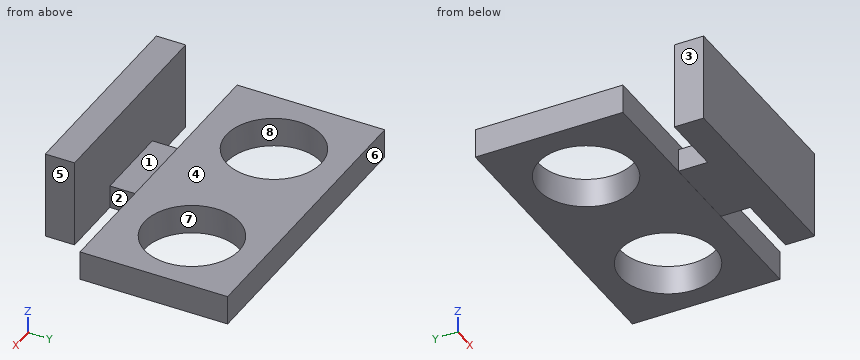
```python
from build123d import *

# Parameters (mm, degrees)
SKETCH1_W           = 35.5
SKETCH1_H           = 15
BOSS_EXTRUDE7_DEPTH = 5
SKETCH5_W           = 13.567085075
SKETCH5_H           = 3.932792286
BOSS_EXTRUDE8_DEPTH = 5
SKETCH6_W           = 50.2
SKETCH6_H           = 5
BOSS_EXTRUDE9_DEPTH = 25.2
SKETCH7_R           = 8.1
CUT_EXTRUDE1_DEPTH  = 10


with BuildPart() as part:
    # Sketch1 → Boss-Extrude7 (new body)
    with BuildSketch(Plane(origin=(0, 0, 0), x_dir=(1, 0, 0), z_dir=(0, 1, 0))):
        with Locations((32.254129859, 13.775388257)):
            Rectangle(SKETCH1_W, SKETCH1_H)
    extrude(amount=BOSS_EXTRUDE7_DEPTH)

    # Sketch5 → Boss-Extrude8 (add)
    with BuildSketch(Plane(origin=(0, 5, 0), x_dir=(1, 0, 0), z_dir=(0, 1, 0))):
        with Locations((31.950040022, 19.308992114)):
            Rectangle(SKETCH5_W, SKETCH5_H)
    extrude(amount=BOSS_EXTRUDE8_DEPTH)

    # Sketch6 → Boss-Extrude9 (add)
    with BuildSketch(Plane(origin=(1.124638213, 10, 0), x_dir=(1, 0, 0), z_dir=(0, 1, 0))):
        with Locations((31.402213384, 18.794771585)):
            Rectangle(SKETCH6_W, SKETCH6_H)
    extrude(amount=BOSS_EXTRUDE9_DEPTH)

    # Sketch7 → Cut-Extrude1 (cut)
    with BuildSketch(Plane.XY.offset(-16.294771585)):
        with Locations((19.758900119, 22.875876323)):
            Circle(SKETCH7_R)
        with Locations((45.958900119, 22.875876323)):
            Circle(SKETCH7_R)
    extrude(amount=-CUT_EXTRUDE1_DEPTH, mode=Mode.SUBTRACT)


solid = part.part
```
Geometry check sheet. Reference: the model listing, model coordinates, mm. Face numbers are marked on the shaded views. A direction names the side the tool comes from. Give positions to 0.01 mm unless a question says otherwise; leave off trailing zeros. Loops run counter-clockwise (first coordinate to the right, second up) from the corner with the lowest first, then second, coordinate; pieces in that order, holes last. Notation, with made-up numbers: M -8,57.5 L -4,57.5 A27 ccw -4,87.5 Z; hole C -15.75,81.5 d1. An arc over 180 degrees is marked long. Write item = value, one per line. Start each with the question number.
1. Section check A-A, the plane y = 30. Enter the section's corners in (x, z), plus the area to 3 significant figures.
2. Section check C-C, the plane x = 22.5. Enter the section's corners in (y, z).
3. Thickness scan on probe 1 along Y at (x, z) = (20, -16.75); probe 2 along Y at (x, z) = (41, -19.5); probe 3 along Y at (x, z) = (38, -7.25). Record the ranges inside material, lowest first.
4. Section check D-D, the plane z = -18. Enter the section's corners in (x, y), plus the area to 3 significant figures.
5. Tool access check on the marked faces 1, 2, 3 and 4. Record the directions out of +Z, -Z, +X, -X, +Y, -Y that give a thin tool (end or side, any length) a straight path to the whole face; none if there is none.
6. Draft check along X on the marked faces 5, 6, 7 and 8. Enter one of: +X half, -X half, draft (parallel to the pull), parting line (faces both ways), or undercut.
7. Go/stop test with flat-tipped pins: P1, Ø4.5, axis at y = 6.5, z = -19.5, coming from the -X side; P2, Ø5.5, axis at y = 2, z = -16.5, coming from the +X side; P3, Ø7.5, axis at x = 37.5, y = 19, coming from the +Z side; P4, Ø2, axis at x = 14.5, y = 9.5, coming from the -Z side. Record where each tip stops, or that it passes through.
8. Section check B-B, the plane x = 13. Enter the section's corners in (y, z).
Values follow:
q1.outline = M 7.43,-21.29 L 15.9,-21.29 L 15.9,-16.29 L 7.43,-16.29 Z; M 23.61,-21.29 L 42.1,-21.29 L 42.1,-16.29 L 23.61,-16.29 Z; M 49.81,-21.29 L 57.63,-21.29 L 57.63,-16.29 L 49.81,-16.29 Z
q1.area = 174 mm^2
q2.outline = M 0,-21.28 L 5,-21.28 L 5,-6.28 L 0,-6.28 Z; M 10,-21.29 L 15.25,-21.29 L 15.25,-16.29 L 10,-16.29 Z; M 30.5,-21.29 L 35.2,-21.29 L 35.2,-16.29 L 30.5,-16.29 Z
q3.probe_1 = 0 to 5, 10 to 14.78, 30.97 to 35.2
q3.probe_2 = 0 to 5, 10 to 16.47, 29.28 to 35.2
q3.probe_3 = 0 to 5
q4.outline = M 7.43,10 L 25.17,10 L 25.17,5 L 14.5,5 L 14.5,0 L 50,0 L 50,5 L 38.73,5 L 38.73,10 L 57.63,10 L 57.63,35.2 L 7.43,35.2 Z; hole C 19.76,22.88 d16.2; hole C 45.96,22.88 d16.2
q4.area = 1,100 mm^2
q5.face_1 = +Z, +X, -X
q5.face_2 = +Z, -Z, +X
q5.face_3 = +Z, -Z, -X, -Y
q5.face_4 = +Z, +X, -X, +Y
q6.face_5 = +X half
q6.face_6 = draft
q6.face_7 = undercut
q6.face_8 = undercut
q7.P1 = 14.5
q7.P2 = 50
q7.P3 = -16.29
q7.P4 = -21.29
q8.outline = M 10,-21.29 L 18.41,-21.29 L 18.41,-16.29 L 10,-16.29 Z; M 27.34,-21.29 L 35.2,-21.29 L 35.2,-16.29 L 27.34,-16.29 Z
